Autodesk Inventor part; units mm, degrees
ref_plane "YZ Plane" through (0, 0, 0) normal (1, 0, 0) x (0, 1, 0)
ref_plane "XZ Plane" through (0, 0, 0) normal (0, 1, 0) x (-1, 0, 0)
ref_plane "XY Plane" through (0, 0, 0) normal (0, 0, 1) x (1, 0, 0)
sketch "Sketch1" plane through (0, 0, 0) normal (0, 1, 0) x (-1, 0, 0)
  arc A0 (0, -177) -> (0, 177) centre (0, 0) ccw
  arc A1 (0, 177) -> (0, -177) centre (0, 0) ccw
  point P0 (-177, 177)
  point P1 (-177, -177)
  dimension "d0" = 354
extrude "Extrusion1" add sketch "Sketch1" along normal blind 5
sketch "Sketch2" plane through (0, 5, 0) normal (0, 1, 0) x (1, 0, 0)
  circle A0 centre (-51.435, -34.125) radius 1.7
  circle A1 centre (-51.435, 34.125) radius 1.7
  circle A2 centre (51.435, 34.125) radius 1.7
  circle A3 centre (51.435, -34.125) radius 1.7
  line L0 (151.6, 177) -> (0, 177) construction
  line L1 (0, -177) -> (0, 177) construction
  circle A4 centre (0, 0) radius 177 construction
  line L2 (-177, 0) -> (177, 0) construction
  circle A5 centre (26.035, 59.5249) radius 1.7
  circle A6 centre (26.035, -59.5249) radius 1.7
  circle A7 centre (-26.035, 59.5249) radius 1.7
  circle A8 centre (-26.035, -59.5249) radius 1.7
  point P0 (177, 177)
  dimension "d5" = 3.4
  dimension "d6" = 3.4
  dimension "d8" = 3.4
  dimension "d10" = 3.4
  dimension "d12" = 68.25
  dimension "d13" = 68.25
  dimension "d14" = 102.87
  dimension "d15" = 102.87
  dimension "d18" = 51.435
  dimension "d19" = 51.435
  dimension "d20" = 34.125
  dimension "d21" = 34.125
  dimension "d153" = 3.4
  dimension "d155" = 3.4
  dimension "d157" = 3.4
  dimension "d159" = 3.4
  dimension "d161" = 52.07
  dimension "d162" = 26.035
  dimension "d163" = 52.07
  dimension "d164" = 26.035
  dimension "d165" = 119.0498
  dimension "d166" = 119.0498
  dimension "d167" = 59.5249
  dimension "d168" = 59.5249
extrude "Jetson Holes" cut sketch "Sketch2" against normal through all
sketch "Sketch3" plane through (0, 5, 0) normal (0, 1, 0) x (1, 0, 0)
  circle A0 centre (-12.7, -63.5) radius 9.525
  circle A1 centre (0, 0) radius 177 construction
  line L0 (151.6, 177) -> (0, 177) construction
  line L1 (-177, 0) -> (0, 0) construction
  line L2 (0, 0) -> (0, -177) construction
  point P0 (177, 177)
  dimension "d24" = 19.05
  dimension "d189" = 63.5
  dimension "d190" = 12.7
extrude "SPI_Holes" cut sketch "Sketch3" against normal through all
sketch "Sketch4" plane through (0, 5, 0) normal (0, 1, 0) x (1, 0, 0)
  circle A0 centre (-60.96, -76.2) radius 1.7
  circle A1 centre (60.96, -101.6) radius 1.7
  circle A2 centre (60.96, 76.2) radius 1.7
  circle A3 centre (-60.96, 101.6) radius 1.7
  line L0 (177, 0) -> (-177, 0) construction
  circle A4 centre (-12.7, -63.5) radius 9.525 construction
  circle A5 centre (-101.6, 50.8) radius 8.89
  circle A6 centre (-101.6, -50.8) radius 8.89
  circle A7 centre (41.91, -76.2) radius 1.7
  circle A8 centre (-41.91, -101.6) radius 1.7
  circle A9 centre (-41.91, 76.2) radius 1.7
  circle A10 centre (41.91, 101.6) radius 1.7
  point P0 (0, 0)
  point P1 (0, -177)
  dimension "d30" = 3.4
  dimension "d31" = 3.4
  dimension "d33" = 3.4
  dimension "d35" = 3.4
  dimension "d37" = 121.92
  dimension "d38" = 121.92
  dimension "d39" = 25.4
  dimension "d40" = 25.4
  dimension "d43" = 12.7
  dimension "d44" = 177.8
  dimension "d45" = 17.78
  dimension "d46" = 17.78
  dimension "d47" = 50.8
  dimension "d48" = 50.8
  dimension "d139" = 3.4
  dimension "d140" = 19.05
  dimension "d141" = 25.4
  dimension "d142" = 3.4
  dimension "d143" = 19.05
  dimension "d144" = 25.4
  dimension "d145" = 3.4
  dimension "d147" = 3.4
  dimension "d149" = 25.4
  dimension "d150" = 25.4
  dimension "d151" = 19.05
  dimension "d152" = 19.05
extrude "NiMH Holes" cut sketch "Sketch4" against normal through all
sketch "Sketch5" plane through (0, 5, 0) normal (0, 1, 0) x (1, 0, 0)
  circle A0 centre (-8.1625, 9.55) radius 1.7
  circle A1 centre (-8.1625, -9.55) radius 1.7
  circle A2 centre (8.1625, -9.55) radius 1.7
  circle A3 centre (8.1625, 9.55) radius 1.7
  line L0 (-177, 0) -> (177, 0)
  line L1 (0, 177) -> (0, -177) construction
  circle A4 centre (0, 0) radius 177 construction
  dimension "d53" = 3.4
  dimension "d54" = 3.4
  dimension "d56" = 3.4
  dimension "d58" = 3.4
  dimension "d60" = 16.325
  dimension "d61" = 16.325
  dimension "d62" = 19.1
  dimension "d63" = 19.1
  dimension "d66" = 9.55
  dimension "d67" = 9.55
  dimension "d191" = 8.1625
  dimension "d192" = 8.1625
extrude "IMU Holes" cut sketch "Sketch5" against normal through all
sketch "Sketch8" plane through (0, 5, 0) normal (0, 1, 0) x (1, 0, 0)
  circle A0 centre (-101.6, 101.6) radius 2.1907
  circle A1 centre (-101.6, -101.6) radius 2.1907
  circle A2 centre (101.6, -101.6) radius 2.1907
  circle A3 centre (101.6, 101.6) radius 2.1907
  line L0 (177, 0) -> (-177, 0) construction
  circle A4 centre (101.6, 0) radius 1.7
  point P0 (0, 0)
  dimension "d97" = 4.3815
  dimension "d98" = 4.3815
  dimension "d100" = 4.3815
  dimension "d102" = 4.3815
  dimension "d105" = 101.6
  dimension "d106" = 101.6
  dimension "d110" = 101.6
  dimension "d111" = 101.6
  dimension "d169" = 3.4
extrude "Level1 Standoffs" cut sketch "Sketch8" against normal through all
sketch "Sketch6" plane through (0, 5, 0) normal (0, 1, 0) x (1, 0, 0)
  circle A0 centre (-82.55, -114.3) radius 1.7
  circle A1 centre (-82.55, 114.3) radius 1.7
  circle A2 centre (82.55, 114.3) radius 1.7
  circle A3 centre (82.55, -114.3) radius 1.7
  point P0 (0, 0)
  point P1 (0, 177)
  dimension "d70" = 3.4
  dimension "d71" = 3.4
  dimension "d73" = 3.4
  dimension "d75" = 3.4
extrude "Level3 Standoffs" cut sketch "Sketch6" against normal through all
sketch "Sketch7" plane through (0, 5, 0) normal (0, 1, 0) x (1, 0, 0)
  line L0 (177, 0) -> (-177, 0) construction
  circle A0 centre (0, 0) radius 177 construction
  circle A1 centre (-141.44, 0) radius 2.667
  circle A2 centre (-114.4274, -83.1363) radius 2.667
  circle A3 centre (-114.4274, 83.1363) radius 2.667
  circle A4 centre (-43.7074, -134.5174) radius 2.667
  circle A5 centre (-43.7074, 134.5174) radius 2.667
  line L1 (0, 177) -> (0, -181.7127) construction
  circle A6 centre (141.44, 0) radius 2.667
  circle A7 centre (114.4274, -83.1363) radius 2.667
  circle A8 centre (114.4274, 83.1363) radius 2.667
  circle A9 centre (43.7074, -134.5174) radius 2.667
  circle A10 centre (43.7074, 134.5174) radius 2.667
  point P0 (-177, 0)
  point P1 (177, 0)
  dimension "d91" = 5.334
  dimension "d92" = 35.56
  dimension "d95" = 144
extrude "Zip Ties" cut sketch "Sketch7" against normal through all
sketch "Sketch9" plane through (0, 5, 0) normal (0, 1, 0) x (1, 0, 0)
  circle A0 centre (-110.89, 17.1) radius 1.7
  circle A1 centre (-110.89, -17.1) radius 1.7
  circle A2 centre (-135.09, 17.1) radius 1.7
  line L0 (0, 0) -> (-177, 0) construction
  circle A3 centre (0, 0) radius 177 construction
  circle A4 centre (-141.44, 0) radius 2.667 construction
  point P0 (0, 177)
  point P1 (0, -177)
  dimension "d171" = 3.4
  dimension "d172" = 3.4
  dimension "d174" = 3.4
  dimension "d176" = 24.2
  dimension "d177" = 34.2
  dimension "d178" = 17.1
  dimension "d179" = 6.35
  dimension "d180" = 17.1
  dimension "d181" = 17.1
extrude "Mic_MCU_Case" cut sketch "Sketch9" against normal blind 25.4
sketch "Sketch12" plane through (0, 5, 0) normal (0, 1, 0) x (1, 0, 0)
  circle A0 centre (31.75, 63.5) radius 1.7
  circle A1 centre (-31.75, 63.5) radius 1.7
  circle A2 centre (-31.75, -63.5) radius 1.7
  circle A3 centre (31.75, -63.5) radius 1.7
  point P0 (0, 0)
  dimension "d193" = 3.4
  dimension "d194" = 3.4
  dimension "d195" = 3.4
  dimension "d196" = 3.4
  dimension "d197" = 63.5
  dimension "d198" = 63.5
  dimension "d199" = 63.5
  dimension "d200" = 63.5
  dimension "d201" = 31.75
  dimension "d202" = 31.75
  dimension "d203" = 31.75
  dimension "d204" = 31.75
extrude "LiDAR Standoffs" cut sketch "Sketch12" against normal blind 25.4
equation "\"d0\" = robot_diameter"
equation "\"d3\" = hardboard_thickness"
equation "\"d5\" = m3_clearance"
equation "\"d6\" = d7"
equation "\"d8\" = d9"
equation "\"d10\" = d11"
equation "\"d13\" = d12"
equation "\"d19\" = d18"
equation "\"d20\" = d21"
equation "\"d21\" = 0.5 * d12"
equation "\"d153\" = d154"
equation "\"d155\" = d156"
equation "\"d157\" = d158"
equation "\"d159\" = d160"
equation "\"d162\" = 0.5 * d161"
equation "\"d163\" = d161"
equation "\"d164\" = d162"
equation "\"d166\" = d165"
equation "\"d167\" = 0.5 * d165"
equation "\"d168\" = d167"
equation "\"d30\" = m3_clearance"
equation "\"d31\" = d32"
equation "\"d33\" = d34"
equation "\"d35\" = d36"
equation "\"d38\" = d37"
equation "\"d40\" = d39"
equation "\"d46\" = d45"
equation "\"d48\" = d47"
equation "\"d139\" = m3_clearance"
equation "\"d141\" = d40"
equation "\"d142\" = m3_clearance"
equation "\"d144\" = d40"
equation "\"d145\" = d146"
equation "\"d147\" = d148"
equation "\"d149\" = d39"
equation "\"d150\" = d39"
equation "\"d152\" = d151"
equation "\"d53\" = m3_clearance"
equation "\"d54\" = d55"
equation "\"d56\" = d57"
equation "\"d58\" = d59"
equation "\"d61\" = d60"
equation "\"d63\" = d62"
equation "\"d66\" = 0.5 * d63"
equation "\"d67\" = d66"
equation "\"d106\" = d105"
equation "\"d110\" = d105"
equation "\"d111\" = d105"
equation "\"d169\" = m3_clearance"
equation "\"d70\" = m3_clearance"
equation "\"d71\" = d72"
equation "\"d73\" = d74"
equation "\"d75\" = d76"
equation "\"d171\" = m3_clearance"
equation "\"d172\" = d173"
equation "\"d174\" = d175"
equation "\"d178\" = 0.5 * d177"
equation "\"d180\" = d178"
equation "\"d181\" = d178"
equation "\"m3_heat_set_insert\" = 4"
equation "\"m3_clearance\" = 3.4"
equation "\"m3_heat_set_depth\" = 7"
equation "\"robot_diameter\" = 354"
equation "\"hardboard_thickness\" = 5"
equation "\"motor_centerline_height\" = 13"
properties part number "layer2"
Geometry: final body of the model. Coordinates: model frame, mm. Give positions to 0.01 mm unless a question says otherwise; leave off trailing zeros. Use CSV: the item, a comma, the result in double quotes.
(1) Ray query, line 1 along Z through (x, y) = (-7.5, 3); line 2 along X through (y, z) = (1.4, 101.6); line 3 along X through (y, z) = (1.35, 135). Return the intervals inside material, ascending. Write a range as [from, to].
From the geometry:
line 1,"[-176.84, -11.12], [-7.98, 7.98], [11.12, 55.52], [71.48, 176.84]"
line 2,"[-144.94, -103.79], [-99.41, -43.61], [-40.21, 59.26], [62.66, 99.41], [103.79, 144.94]"
line 3,"[-114.47, -46.33], [-41.08, 41.08], [46.33, 114.47]"
(2) First-contact query: P1, Ø1.5, axis at y = 1, z = 12.5, coming from the +X side; P2, Ø1, axis at x = 15.5, y = 3.5, coming from the -Z side; P3, Ø1.5, axis at x = -19.5, y = 3, coming from the +Z side. Flat tips, straight axial feed; report the tip coordinate or a pass-through.
From the geometry:
P1,"x = 176.61"
P2,"z = -176.36"
P3,"z = 176"
(3) Pull-direction query (X, two-part tool) for faces 1 (the face through (2, 5, 2)), 2 (the face through (172.79, 2.46, -38.37)), 3 (the face through (-110.48, 2.54, -51.19)); classes: released by +X, released by -X, zero draft, split by the parting line, or undercut.
From the geometry:
face 1,"zero draft"
face 2,"split by the parting line"
face 3,"undercut"
(4) Cut plane A-A (y = 2.95). Count the separate pieces of the cut face and the enclosed holes in it, plus the area to 3 significant figures.
From the geometry:
separate pieces,"1"
enclosed holes,"49"
area,"97,100 mm^2"
